Design review of the part built by this model. Coordinates are the model's own, in mm. Give positions to 0.01 mm unless a question says otherwise; leave off trailing zeros. Order: outer loops, then holes, each group sorted by start corner. A loop starts at its lowest first (then second) coordinate and runs counter-clockwise, first axis right, second up. Notation, with made-up numbers: (44.25, 15) -> (49.25, 15) arc R11 ccw to (49.25, 24) -> close; hole circle Ø9 at (77, 21.25). An arc over 180 degrees is marked (long way). Return JSON: item names as keys, results as strings.
Autodesk Inventor part; units mm, degrees
ref_plane "YZ Plane" through (0, 0, 0) normal (1, 0, 0) x (0, 1, 0)
ref_plane "XZ Plane" through (0, 0, 0) normal (0, 1, 0) x (-1, 0, 0)
ref_plane "XY Plane" through (0, 0, 0) normal (0, 0, 1) x (1, 0, 0)
sketch "Sketch1" plane through (0, 0, 0) normal (0, 0, 1) x (1, 0, 0)
  line L0 (350, -136.5) -> (-350, -136.5)
  line L1 (-350, -136.5) -> (-350, 136.5)
  line L2 (-350, 136.5) -> (350, 136.5)
  line L3 (350, 136.5) -> (350, -136.5)
  line L4 (350, -136.5) -> (-350, 136.5) construction
  line L5 (-350, -136.5) -> (350, 136.5) construction
  point P0 (0, 0)
  dimension "d0" = 273
  dimension "d1" = 700
extrude "Extrusion1" add sketch "Sketch1" along normal blind 3
sketch "Sketch5" plane through (0, 0, 3) normal (0, 0, 1) x (1, 0, 0)
  line L0 (-300, 84.5) -> (-175, 84.5)
  line L1 (-175, 84.5) -> (-175, 96.5)
  line L2 (-175, 96.5) -> (-300, 96.5)
  line L3 (-300, 96.5) -> (-300, 84.5)
  line L4 (-62.5, 96.5) -> (62.5, 96.5)
  line L5 (62.5, 96.5) -> (62.5, 84.5)
  line L6 (62.5, 84.5) -> (-62.5, 84.5)
  line L7 (-62.5, 84.5) -> (-62.5, 96.5)
  line L8 (350, 136.5) -> (-350, 136.5)
  line L9 (175, 84.5) -> (300, 84.5)
  line L10 (300, 84.5) -> (300, 96.5)
  line L11 (300, 96.5) -> (175, 96.5)
  line L12 (175, 96.5) -> (175, 84.5)
  line L13 (-350, 136.5) -> (-350, -136.5)
  point P0 (0, 0)
  dimension "d21" = 12
  dimension "d29" = 40
  dimension "d30" = 40
  dimension "d33" = 40
  dimension "d35" = 50
  dimension "d36" = 50
  dimension "d37" = 112.5
  dimension "d38" = 112.5
  dimension "d41" = 12
  dimension "d42" = 12
extrude "Extrusion5" cut sketch "Sketch5" against normal blind 10
fillet "Fillet5" radius 6 4 edges at (-300, 96.5, 1.5) (-300, 84.5, 1.5) (-175, 84.5, 1.5) (-175, 96.5, 1.5)
fillet "Fillet6" radius 6 8 edges at (-62.5, 96.5, 1.5) (-62.5, 84.5, 1.5) (62.5, 96.5, 1.5) (62.5, 84.5, 1.5) (175, 96.5, 1.5) (175, 84.5, 1.5) (300, 96.5, 1.5) (300, 84.5, 1.5)
equation "\"d30\" = d29"
equation "\"d33\" = d29"
equation "\"d41\" = d21"
equation "\"d42\" = d21"
equation "\"d40\" = 0.5 * d21"
equation "\"d43\" = 0.5 * d21"
properties part number "GBX_021.1-front-PMMA"
Item 1: Add section A-A (x = 3). Give the boundary of the cut face in (y, z), plus the area to 3 significant figures.
Result set:
{"outline": "(-136.5, 0) -> (84.5, 0) -> (84.5, 3) -> (-136.5, 3) -> close; (96.5, 0) -> (136.5, 0) -> (136.5, 3) -> (96.5, 3) -> close", "area": "783 mm^2"}
Item 2: For pin 1 (4 mm diameter, centred on x = -6.5, y = 93, fed in from -Z), flat-tipped, find the tip position at first contact; note if it passes through.
Result set:
{"pin 1": "passes through"}
Item 3: Wall thickness on L1, parallel to X at y = 91, z = 1.9; L2, parallel to Y at x = 24.5, z = 1.3: over which ranges is each line inside the solid? List them lowest first. Write a range as [from, to].
Result set:
{"L1": "x = [-350, -299.98], [-175.02, -62.48], [62.48, 175.02], [299.98, 350]", "L2": "y = [-136.5, 84.5], [96.5, 136.5]"}
Item 4: Add section B-B (z = 1.45). Give the number of separate pieces and of enclosed holes in the cut face, plus the area to 3 significant figures.
Result set:
{"separate pieces": "1", "enclosed holes": "3", "area": "187,000 mm^2"}
